For this review, take the finished solid that the model builds, in its own axes (mm). Face numbers are marked on the shaded views. A direction names the side the tool comes from. Coordinates: 2 decimals unless noted, no trailing zeros. Order: outer loops, then holes, each group sorted by start corner. A loop starts at its lowest first (then second) coordinate and runs counter-clockwise, first axis right, second up. Notation, with made-up numbers: (56, 81) -> (111, 81) arc R23 ccw to (111, 118) -> close; hole circle Ø7 at (19, 4.5). An arc over 180 degrees is marked (long way). Answer as a JSON object with one key per item and string values. Group by question number.
1) For pin 1 (2.5 mm diameter, centred on x = 10, y = 8, fed in from -Z); pin 2 (3.5 mm diameter, centred on y = 7.5, z = -5, fed in from -X); pin 3 (6 mm diameter, centred on x = -35, y = 7.5, fed in from +Z), all flat-tipped, find the tip position at first contact; note any pin that passes through.
2) Machinability: for the marked faces 4, 5 and 6, which of the approach directions +Z, -Z, +X, -X, +Y, -Y give a long, thin tool a straight path to every point of the face, cutting with its end or side? Answer none if there is none.
3) Wall thickness on L1, parallel to X at y = 11, z = -10.25; L2, parallel to X at y = 6.25, z = -6.5; L3, parallel to Y at x = -31, z = -5: over which ranges is each line inside the solid? List them lowest first.
4) Add section A-A, the plane z = -8.75. Count the separate pieces of the cut face and the enclosed holes in it, then the cut area to 3 significant figures.
5) Add section C-C, the plane x = -7. Write out the cut boundary in (y, z), then the cut area to 3 significant figures.
6) Draft analysis for pull direction X (two halves, no side actions). For the marked faces 1, 2 and 3, state which applies: +X half, -X half, draft (parallel to the pull), parting line (faces both ways), or undercut.
7) Add section B-B, the plane x = -38. Write out the cut boundary in (y, z), then the cut area to 3 significant figures.
Solid Edge part; units mm, degrees
sketch "Sketch1" plane through (0, 0, 0) normal (0, -1, 0) x (1, 0, 0)
  line L0 (-33, -12.5) -> (33, -12.5)
  line L1 (33, -12.5) -> (33, 12.5)
  line L2 (33, 12.5) -> (-33, 12.5)
  line L3 (-33, 12.5) -> (-33, -12.5)
  dimension "D1" = 33
  dimension "D2" = 33
extrude "Protrusion1" add sketch "Sketch1" against normal blind 12
sketch "Sketch2" plane through (0, 6, -12.5) normal (0, 0, -1) x (1, 0, 0)
  line L0 (13, 6) -> (13, -6)
  line L1 (13, -6) -> (23, -6)
  line L2 (23, 6) -> (23, -6)
  line L3 (13, 6) -> (23, 6)
  line L4 (-5, 6) -> (5, 6)
  line L5 (5, 6) -> (5, -6)
  line L6 (5, -6) -> (-5, -6)
  line L7 (-5, -6) -> (-5, 6)
  line L8 (-23, 6) -> (-23, -6)
  line L9 (-23, -6) -> (-13, -6)
  line L10 (-13, 6) -> (-13, -6)
  line L11 (-23, 6) -> (-13, 6)
  dimension "D1" = 5
extrude "Extrusionsausschnitt_1" cut sketch "Sketch2" against normal blind 20
sketch "Sketch3" plane through (-33, 6, 0) normal (-1, 0, 0) x (0, -1, 0)
  line L0 (-6, 12.5) -> (6, 12.5)
  line L1 (6, 12.5) -> (6, -2.5)
  line L2 (6, -2.5) -> (-6, -2.5)
  line L3 (-6, -2.5) -> (-6, 12.5)
extrude "Extrusionsausprägung_2" add sketch "Sketch3" along normal blind 20
mirror "Mirror1" about plane through (0, 0, 0) normal (1, 0, 0) of "Extrusionsausprägung_2"
sketch "Sketch4" plane through (0, 0, 0) normal (0, -1, 0) x (1, 0, 0)
  line L0 (-33, -10.5) -> (33, -10.5)
extrude "Extrusionsausschnitt_3" cut sketch "Sketch4" against normal blind 62.4108 material side at (0, 0, -10.55)
sketch "Sketch5" plane through (0, 0, 1) normal (0, -1, 0) x (1, 0, 0)
  line L0 (-53, 1.5) -> (-33, 1.5)
  line L1 (-33, 1.5) -> (-23, 11.5)
  dimension "D1" = 53
extrude "Extrusionsausschnitt_4" cut sketch "Sketch5" against normal blind 64.7066 material side at (-43, 0, 2.55)
hole "Bohrung_1" at (-48, 6, 2.5) direction (0, 0, -1) diameter 5.8 end up to next
hole "Hole1" at (-38, 6, 2.5) direction (0, 0, -1) diameter 5.8 end up to next
fillet "Verrundung_1" radius 0.5 2 edges at (-33, 6, 2.5) (-23, 6, 12.5)
chamfer "Fase_1" distance 1 angle 45 4 edges at (-23, 6, 7.5) (-13, 6, 7.5) (13, 6, 7.5) (23, 6, 7.5)
mirror "Mirror2" about plane through (0, 0, 0) normal (1, 0, 0) of "Extrusionsausschnitt_4", "Bohrung_1", "Hole1"
fillet "Round1" radius 0.5 2 edges at (33, 6, 2.5) (23, 6, 12.5)
chamfer "Chamfer1" [suppressed]
sketch "Sketch6" plane through (43.1036, 6, 2.5) normal (0, 0, 1) x (1, 0, 0)
  line L0 (-0.1036, 6) -> (-0.1036, -6)
extrude "Extrusionsausschnitt_6" cut sketch "Sketch6" against normal blind 27.3244 material side at (43.05, 6, 2.5)
chamfer "Fase_3" distance 1 angle 45 2 edges at (-5, 6, 7.5) (5, 6, 7.5)
sketch "Sketch7" plane through (-5, 0, 1) normal (0, -1, 0) x (1, 0, 0)
  line L0 (-28, -7.6) -> (-48, -7.6)
  line L1 (-48, -7.6) -> (-48, -12.6)
  line L2 (-48, -12.6) -> (-18, -12.6)
  line L3 (-18, -12.6) -> (-18, -11.5)
  line L4 (-18, -11.5) -> (-28, -11.5)
  line L5 (-28, -11.5) -> (-28, -7.6)
  line L6 (38, -7.6) -> (48, -7.6)
  line L7 (48, -7.6) -> (48, -12.6)
  line L8 (48, -12.6) -> (28, -12.6)
  line L9 (28, -12.6) -> (28, -11.5)
  line L10 (28, -11.5) -> (38, -11.5)
  line L11 (38, -11.5) -> (38, -7.6)
  line L12 (-8, -11.5) -> (0, -11.5)
  line L13 (0, -11.5) -> (0, -12.5024)
  line L14 (0, -12.5024) -> (-8, -12.5024)
  line L15 (-8, -12.5024) -> (-8, -11.5)
  line L16 (10, -11.5) -> (18, -11.5)
  line L17 (18, -11.5) -> (18, -12.5)
  line L18 (18, -12.5) -> (10, -12.5)
  line L19 (10, -12.5) -> (10, -11.5)
  dimension "D1" = 48
  dimension "D2" = 48
  dimension "D3" = 18
extrude "Protrusion3" add sketch "Sketch7" against normal up to vertex (12 mm away)
sketch "Sketch8" plane through (-38, 6, -11.6) normal (0, 0, -1) x (1, 0, 0)
  line L0 (-12.225, 3.8538) -> (-14.45, 0)
  line L1 (-14.45, 0) -> (-12.225, -3.8538)
  line L2 (-12.225, -3.8538) -> (-7.775, -3.8538)
  line L3 (-7.775, -3.8538) -> (-5.55, 0)
  line L4 (-5.55, 0) -> (-7.775, 3.8538)
  line L5 (-7.775, 3.8538) -> (-12.225, 3.8538)
  line L6 (-2.225, 3.8538) -> (-4.45, 0)
  line L7 (-4.45, 0) -> (-2.225, -3.8538)
  line L8 (-2.225, -3.8538) -> (2.225, -3.8538)
  line L9 (2.225, -3.8538) -> (4.45, 0)
  line L10 (4.45, 0) -> (2.225, 3.8538)
  line L11 (2.225, 3.8538) -> (-2.225, 3.8538)
  line L12 (73.775, 3.8538) -> (71.55, 0)
  line L13 (71.55, 0) -> (73.775, -3.8538)
  line L14 (73.775, -3.8538) -> (78.225, -3.8538)
  line L15 (78.225, -3.8538) -> (80.45, 0)
  line L16 (80.45, 0) -> (78.225, 3.8538)
  line L17 (78.225, 3.8538) -> (73.775, 3.8538)
extrude "Cutout2" cut sketch "Sketch8" against normal blind 5
sketch "Sketch9" plane through (-33, 6, -3) normal (-1, 0, 0) x (0, -1, 0)
  circle A0 centre (-2, -2) radius 2.05
extrude "Cutout3" cut sketch "Sketch9" along normal up to vertex (20 mm away) and the other way up to vertex (76 mm away)
properties part number "6" material "Polykarbonat"
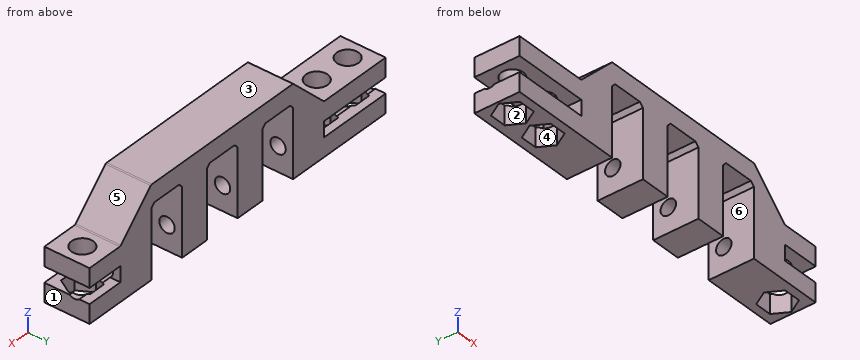
Output values:
{
 "1": {"pin 1": "stops at z = -11.5", "pin 2": "stops at x = -33", "pin 3": "stops at z = 3.5"},
 "2": {"face 4": "-Z", "face 5": "+Z, +X, +Y, -Y", "face 6": "-Z, +Y, -Y"},
 "3": {"L1": "x = -53 to -23, -13 to -5, 5 to 13, 23 to 43", "L2": "x = -33 to -23, -13 to -5, 5 to 13, 23 to 33", "L3": "y = 0 to 5.95, 10.05 to 12"},
 "4": {"separate pieces": "4", "enclosed holes": "3", "area": "638 mm²"},
 "5": {"outline": "(0, -11.5) -> (12, -11.5) -> (12, 12.5) -> (0, 12.5) -> close; hole circle Ø4.1 at (8, -5)", "area": "275 mm²"},
 "6": {"face 1": "+X half", "face 2": "undercut", "face 3": "draft"},
 "7": {"outline": "(0, -11.6) -> (2.15, -11.6) -> (2.15, -6.6) -> (0, -6.6) -> close; (0, -2.5) -> (3.1, -2.5) -> (3.1, 2.5) -> (0, 2.5) -> close; (8.9, -2.5) -> (12, -2.5) -> (12, 2.5) -> (8.9, 2.5) -> close; (9.85, -11.6) -> (12, -11.6) -> (12, -6.6) -> (9.85, -6.6) -> close", "area": "52.5 mm²"}
}
